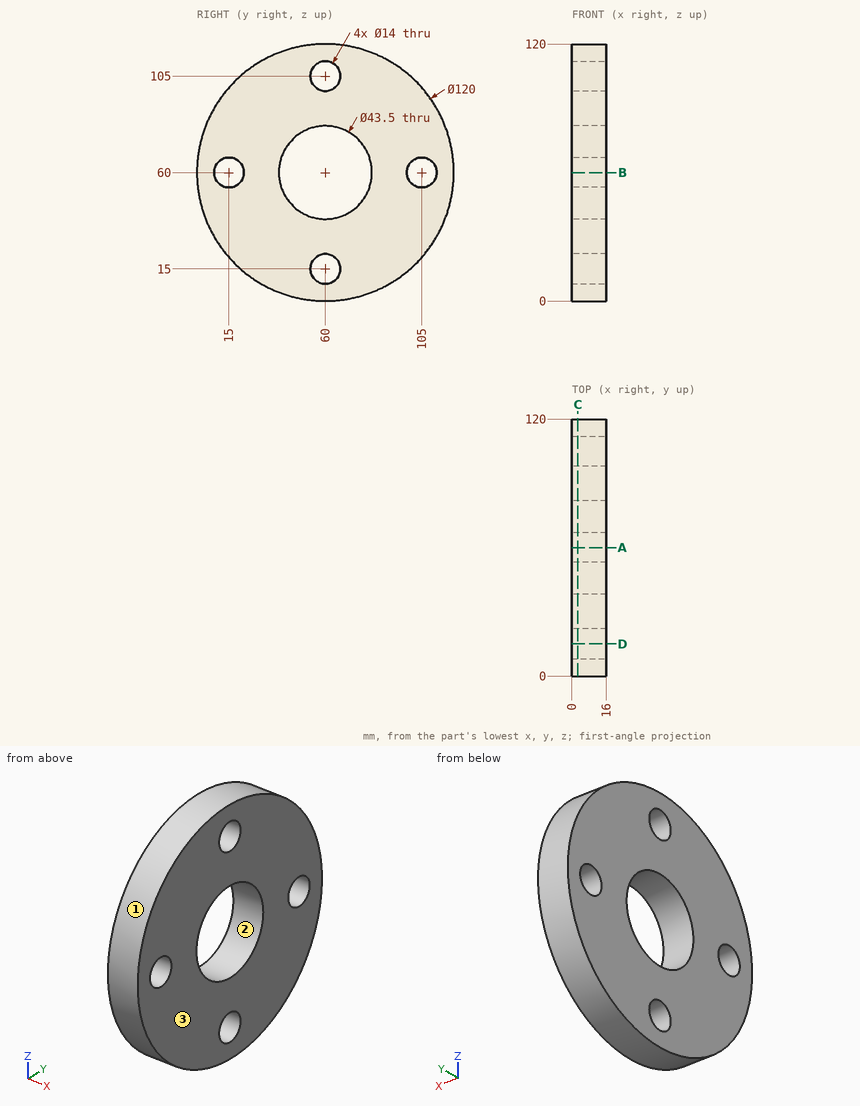
Print and shaded views of the part. All mm, measured from the part's lowest x, y and z. Round coordinates to 2 decimals unless told otherwise and drop trailing zeros. Write each loop counter-clockwise with the first axis right and the second up, starting at its lowest first coordinate (ties: lowest second). Pieces come first, ordered by that corner, then holes. Notation, with made-up numbers: (4, 70) -> (54, 70) arc R20 ccw to (54, 89) -> close; hole circle Ø3 at (60, 17.5). An arc over 180 degrees is marked (long way). Answer in a Markdown table with one row per item. Add a question column.
Item 1: Saw through at D-D, the plane y = 15. Write the cut outline in (x, z), then the cut area to 3 significant figures.
Item 2: Drill centre lines: line 1 (Z direction, x = 3.75, y = 60); line 2 (Z direction, x = 7.25, y = 59); line 3 (Z direction, x = 2.5, y = 80). Where is each one in solid material? Low to high. Write a range as from..to.
Item 3: Saw through at A-A, the plane y = 60. Write the cut outline in (x, z), then the cut area to 3 significant figures.
Item 4: Saw through at C-C, the plane x = 2.75. Write the cut outline in (y, z), then the cut area to 3 significant figures.
Item 5: Drop flat-ended pins along their axis: pin 1 Ø12.5 at (y, z) = (60, 105) entering from -X (3 decimals); pin 2 Ø8 at (x, z) = (2, 91.5) entering from +Y; pin 3 Ø1 at (x, y) = (10.5, 94.5) entering from -Z; pin 4 Ø1 at (x, y) = (11, 92) entering from -Z. Give the stop position or say it passes through.
Item 6: Mould opens along Y. For the marked faces 1, 2 and 3 say: pulls with the +Y half, pulls with the -Y half, needs draft (parallel to the pull), parting line crosses it, or undercut.
Findings below:
| question | item | result |
|---|---|---|
| 1 | outline | (0, 20.31) -> (16, 20.31) -> (16, 53) -> (0, 53) -> close; (0, 67) -> (16, 67) -> (16, 99.69) -> (0, 99.69) -> close |
| 1 | area | 1,050 mm^2 |
| 2 | line 1 | z = 0..8, 22..38.25, 81.75..98, 112..120 |
| 2 | line 2 | z = 0.01..8.07, 21.93..38.27, 81.73..98.07, 111.93..119.99 |
| 2 | line 3 | z = 3.43..51.45, 68.55..116.57 |
| 3 | outline | (0, 0) -> (16, 0) -> (16, 8) -> (0, 8) -> close; (0, 22) -> (16, 22) -> (16, 38.25) -> (0, 38.25) -> close; (0, 81.75) -> (16, 81.75) -> (16, 98) -> (0, 98) -> close; (0, 112) -> (16, 112) -> (16, 120) -> (0, 120) -> close |
| 3 | area | 776 mm^2 |
| 4 | outline | circle Ø120 at (60, 60); hole circle Ø14 at (15, 60); hole circle Ø43.5 at (60, 60); hole circle Ø14 at (60, 15); hole circle Ø14 at (60, 105); hole circle Ø14 at (105, 60) |
| 4 | area | 9,210 mm^2 |
| 5 | pin 1 | passes through |
| 5 | pin 2 | stops at y = 113.33 |
| 5 | pin 3 | stops at z = 10.56 |
| 5 | pin 4 | stops at z = 8.93 |
| 6 | face 1 | parting line crosses it |
| 6 | face 2 | undercut |
| 6 | face 3 | needs draft |
